Can you work these out from the model? Positions are in its coordinate system, mm. A direction names the side the tool comes from. Round coordinates to 2 decimals unless told otherwise and drop trailing zeros. Loops run counter-clockwise (first coordinate to the right, second up) from the corner with the lowest first, then second, coordinate; pieces in that order, holes last. Notation, with made-up numbers: (13.5, 84.5) -> (37.5, 84.5) arc R8 cw to (37.5, 96.5) -> close; hole circle Ø3 at (24, -23.75). An arc over 180 degrees is marked (long way). Use a Markdown table: item, result.
from build123d import *

# Parameters (mm, degrees)
F0_R     = 1.5
F1_DEPTH = 7.5
F2_R     = 1.5
F3_DEPTH = 5
F4_R     = 2.4999


# Not quite as in the source:
# - a fillet or chamfer is up to 0.001 mm smaller than in the source, because OpenCascade refuses the exact size
# - a pattern or mirror of a feature is missing from the dataset's text; its kind, count and spacing are read off the source's solid


with BuildPart() as f1:
    # F0 (on Right) → F1 (new body, symmetric)
    with BuildSketch(Plane.YZ):
        with BuildLine():
            Line((-4.5, -0.685833849), (-2.5, -0.685833849))
            Line((-2.5, -0.685833849), (2.5, -0.685833849))
            Line((2.5, -0.685833849), (2.5, 8.314166151))
            ThreePointArc((2.5, 8.314166151), (0, 10.814166151), (-2.5, 8.314166151))
            Line((-2.5, 8.314166151), (-2.5, 6.314166151))
            ThreePointArc((-2.5, 6.314166151), (-3.0857864376, 4.8999525886), (-4.5, 4.314166151))
            ThreePointArc((-4.5, 4.314166151), (-7, 1.814166151), (-4.5, -0.685833849))
        make_face()
        with Locations((0, 8.314166151)):
            Circle(F0_R, mode=Mode.SUBTRACT)
    extrude(amount=F1_DEPTH, both=True)

    # F2 (on face) → F3 (join)
    with BuildSketch(Plane.YZ.offset(7.5)):
        with BuildLine():
            Line((-17.5, -0.685833849), (0, -0.685833849))
            ThreePointArc((0, -0.685833849), (2.5, 1.814166151), (0, 4.314166151))
            Line((0, 4.314166151), (-17.5, 4.314166151))
            ThreePointArc((-17.5, 4.314166151), (-20, 1.814166151), (-17.5, -0.685833849))
        make_face()
        with Locations((-17.5, 1.814166151)):
            Circle(F2_R, mode=Mode.SUBTRACT)
    f3 = extrude(amount=F3_DEPTH)

    # F3_copies: F3 across plane
    add(f3.mirror(Plane(origin=(0, 0, 0), x_dir=(0, 0, -1), z_dir=(-1, 0, 0))))

    # F4 (radius 2.5 in the source; OpenCascade refuses exactly that, so slightly less here)
    f4_edges = [f1.edges().sort_by_distance(p)[0] for p in [
        (0, 2.5, -0.685834),
    ]]
    fillet(f4_edges, radius=F4_R)


solid = f1.part
1. I want a section at C-C (z = 7.25). Please give me the cut outline in (x, y), plus the area to 3 significant figures.
Answer sheet:
| item | result |
|---|---|
| outline | (-7.5, -2.5) -> (7.5, -2.5) -> (7.5, -1.06) -> (-7.5, -1.06) -> close; (-7.5, 1.06) -> (7.5, 1.06) -> (7.5, 2.5) -> (-7.5, 2.5) -> close |
| area | 43.3 mm² |
2. I want a section at D-D (y = -3.25). Please give me the cut outline in (x, z), plus the area to 3 significant figures.
Answer sheet:
| item | result |
|---|---|
| outline | (-12.5, -0.69) -> (12.5, -0.69) -> (12.5, 4.31) -> (7.5, 4.31) -> (7.5, 4.75) -> (-7.5, 4.75) -> (-7.5, 4.31) -> (-12.5, 4.31) -> close |
| area | 132 mm² |
3. Will these pins go through, and if not, where does the flat tip stop? pin 1 Ø5.5 at (x, y) = (-9, -6) entering from +Z; pin 2 Ø4 at (x, y) = (10.5, -6.5) entering from +Z; pin 3 Ø2 at (y, z) = (0.5, 7) entering from -X; pin 4 Ø2.5 at (y, z) = (-17.5, 1.81) entering from +X.
Answer sheet:
| item | result |
|---|---|
| pin 1 | stops at z = 4.48 |
| pin 2 | stops at z = 4.31 |
| pin 3 | stops at x = -7.5 |
| pin 4 | passes through |
4. If we mould it in two halves opening along Z, with no side actions, what happens to faces 1 (the cylindrical face through (9.96, -19, 1.88)), 2 (the cylindrical face through (-10, -20, 1.9)), 3 (the flat face through (0, 2.5, 5)), 4 (the cylindrical face through (-0.11, -0.33, 6.85))? For each: +Z half, -Z half, draft (parallel to the pull), parting line (faces both ways), or undercut.
Answer sheet:
| item | result |
|---|---|
| face 1 | undercut |
| face 2 | parting line |
| face 3 | draft |
| face 4 | undercut |
5. I want a section at B-B (x = -3.5). Please give me the cut outline in (y, z).
Answer sheet:
| item | result |
|---|---|
| outline | (-4.5, -0.69) -> (0, -0.69) arc R2.5 ccw to (2.5, 1.81) -> (2.5, 8.31) arc R2.5 ccw to (-2.5, 8.31) -> (-2.5, 6.31) arc R2 cw to (-4.5, 4.31) arc R2.5 ccw to start; hole circle Ø3 at (0, 8.31) |
6. Which directions (+Z, -Z, +X, -X, +Y, -Y) give clear straight access to the entire face, cutting with the end or side of a thin tool? Please do faces 5 (the cylindrical face through (10, 2.5, 1.8)), 6 (the cylindrical face through (10, -20, 1.9)), 7 (the flat face through (0, -2.5, 7)).
Answer sheet:
| item | result |
|---|---|
| face 5 | +X, +Y |
| face 6 | +X, -X, -Y |
| face 7 | +Z, +X, -X, -Y |
7. I need wall thicknesses on line 1 (X direction, y = -11, z = 4.25); line 2 (Z direction, x = -2, y = 0); line 3 (Z direction, x = -8.55, y = -17.5). Which ranges of each line are inside material? Lowest first, please.
Answer sheet:
| item | result |
|---|---|
| line 1 | x = -12.5 to -7.5, 7.5 to 12.5 |
| line 2 | z = -0.69 to 6.81, 9.81 to 10.81 |
| line 3 | z = -0.69 to 0.31, 3.31 to 4.31 |
8. I want a section at A-A (y = -13.5). Please give me the cut outline in (x, z).
Answer sheet:
| item | result |
|---|---|
| outline | (-12.5, -0.69) -> (-7.5, -0.69) -> (-7.5, 4.31) -> (-12.5, 4.31) -> close; (7.5, -0.69) -> (12.5, -0.69) -> (12.5, 4.31) -> (7.5, 4.31) -> close |
